Design review of the part built by this model. Coordinates are the model's own, in mm. A direction names the side the tool comes from. Give positions to 0.01 mm unless a question says otherwise; leave off trailing zeros. Write each loop counter-clockwise with the first axis right and the second up, starting at its lowest first coordinate (ties: lowest second). Pieces come first, ordered by that corner, then holes. Notation, with made-up numbers: (-32.75, 88) -> (-15.75, 88) arc R21 ccw to (-15.75, 110) -> close; hole circle Ø11 at (17.25, 76). An arc over 180 degrees is marked (long way). Write each question's results on one line, items separated by ' | '. Start each with the question number.
(1) To check wall thickness, follow probe 1 along Y at (x, z) = (81.5, 1.1); probe 2 along Y at (x, z) = (63.5, 2.95); probe 3 along X at (y, z) = (-4, 1.3) (3 decimals). State the ranges of each line that lie inside material, in increasing order.
(2) Take a section at A-A (y = 56). State the section outline as (x, z) points.
(3) Clearance check with flat-ended pins moving along their axes: pin 1 (1.2 mm diameter, centred on y = -0.5, z = 2, fed in from +X); pin 2 (2 mm diameter, centred on y = 26.5, z = 2, fed in from -X); pin 3 (1 mm diameter, centred on x = 41, y = 82.5, fed in from -Z); pin 4 (1.2 mm diameter, centred on x = 41.5, z = 2, fed in from -Y). State where each tip first meets the part, or that it passes through.
(4) Take a section at B-B (x = 53). State the section outline as (y, z) points, plus the area to 3 significant figures.
(5) For faces 1 (the face through (99.203, 19, 2)), 2 (the face through (-51.35, -42.92, 1.97)), list the 3-axis set-ups (+Z, -Z, +X, -X, +Y, -Y) from which the entire face can be reached by the end or side of a thin tool; tool diameter is ignored.
from build123d import *

# Parameters (mm, degrees)
F1_DEPTH = 4


with BuildPart() as f1:
    # F0 (on Top) → F1 (new body)
    with BuildSketch(Plane.XY):
        with BuildLine():
            Line((99.202662, 19.896773), (99.202662, 83.293949))
            ThreePointArc((99.202662, 83.293949), (102.639271, 102.736338), (83.237467, 99.077547))
            Line((83.237467, 99.077547), (19.823141, 99.077547))
            Line((19.823141, 99.077547), (-43.277989, 98.971398))
            ThreePointArc((-43.277989, 98.971398), (-62.685056, 102.776986), (-59.289763, 83.293949))
            Line((-59.289763, 83.293949), (-59.289763, 19.831447))
            Line((-59.289763, 19.831447), (-59.289763, -43.656712))
            ThreePointArc((-59.289763, -43.656712), (-62.72245, -63.080861), (-43.329186, -59.477778))
            Line((-43.329186, -59.477778), (83.190888, -59.221403))
            ThreePointArc((83.190888, -59.221403), (102.597955, -63.026992), (99.202662, -43.543955))
            Line((99.202662, -43.543955), (99.202662, 19.853222))
            Line((99.202662, 19.853222), (99.202662, 19.896773))
        make_face()
        with BuildLine():
            ThreePointArc((-42.274781, -54.475997), (-42.640605, -51.616895), (-43.677664, -48.927507))
            Line((-43.677664, -48.927507), (-24.605699, -29.855542))
            Line((-24.605699, -29.855542), (10.1243, -48.890038))
            Line((10.1243, -48.890038), (15.366075, -54.379034))
            Line((15.366075, -54.379034), (-42.274781, -54.475997))
        make_face(mode=Mode.SUBTRACT)
        with BuildLine():
            Line((-29.65462, -24.938536), (-48.66586, -43.949777))
            ThreePointArc((-48.66586, -43.949777), (-51.392585, -42.909613), (-54.289763, -42.558424))
            Line((-54.289763, -42.558424), (-54.289763, -42.539768))
            Line((-54.289763, -42.539768), (-54.289763, 15.079639))
            Line((-54.289763, 15.079639), (-48.808765, 9.87071))
            Line((-48.808765, 9.87071), (-29.65462, -24.938536))
        make_face(mode=Mode.SUBTRACT)
        with BuildLine():
            Line((20.115596, -48.890038), (-21.068434, -26.318277))
            Line((-21.068434, -26.318277), (0.785377, -4.464466))
            ThreePointArc((0.785377, -4.464466), (2.407493, -3.380602), (4.320911, -3))
            Line((4.320911, -3), (35.678927, -3))
            ThreePointArc((35.678927, -3), (37.592344, -3.380602), (39.214461, -4.464466))
            Line((39.214461, -4.464466), (61.034324, -26.284329))
            Line((61.034324, -26.284329), (20.115596, -48.890038))
        make_face(mode=Mode.SUBTRACT)
        with BuildLine():
            Line((64.568139, -29.818144), (83.594024, -48.844029))
            ThreePointArc((83.594024, -48.844029), (82.583872, -51.452044), (82.204858, -54.223054))
            Line((82.204858, -54.223054), (24.869697, -54.363046))
            Line((24.869697, -54.363046), (30.045989, -48.890038))
            Line((30.045989, -48.890038), (64.568139, -29.818144))
        make_face(mode=Mode.SUBTRACT)
        with BuildLine():
            Line((20.061165, 4.731285), (20.02865, 4.750027))
            ThreePointArc((20.02865, 4.750027), (20.061339, 4.750123), (20.094027, 4.75029))
            Line((20.094027, 4.75029), (20.061165, 4.731285))
        make_face(mode=Mode.SUBTRACT)
        with BuildLine():
            ThreePointArc((94.058243, -42.453536), (91.243307, -42.823298), (88.594024, -43.844029))
            Line((88.594024, -43.844029), (69.601331, -24.851336))
            Line((69.601331, -24.851336), (88.739303, 9.928519))
            Line((88.739303, 9.928519), (94.211702, 15.119198))
            Line((94.211702, 15.119198), (94.058243, -42.453536))
        make_face(mode=Mode.SUBTRACT)
        with BuildLine():
            Line((-8.87868, -3.300258), (-26.42517, -20.846748))
            Line((-26.42517, -20.846748), (-48.808765, 19.831447))
            Line((-48.808765, 19.831447), (-26.131123, 61.044022))
            Line((-26.131123, 61.044022), (-9.464466, 44.377365))
            ThreePointArc((-9.464466, 44.377365), (-8.380602, 42.755248), (-8, 40.841831))
            Line((-8, 40.841831), (-8, -1.178937))
            ThreePointArc((-8, -1.178937), (-8.228361, -2.326988), (-8.87868, -3.300258))
        make_face(mode=Mode.SUBTRACT)
        with BuildLine():
            Line((-48.681125, 83.594024), (-29.666657, 64.579555))
            Line((-29.666657, 64.579555), (-48.808765, 29.792184))
            Line((-48.808765, 29.792184), (-54.289763, 24.583255))
            Line((-54.289763, 24.583255), (-54.289763, 82.202662))
            ThreePointArc((-54.289763, 82.202662), (-51.400442, 82.555695), (-48.681125, 83.594024))
        make_face(mode=Mode.SUBTRACT)
        with BuildLine():
            Line((9.91038, 88.596564), (-24.61177, 69.524669))
            Line((-24.61177, 69.524669), (-43.681125, 88.594024))
            ThreePointArc((-43.681125, 88.594024), (-42.670973, 91.202039), (-42.291959, 93.973049))
            Line((-42.291959, 93.973049), (15.086671, 94.069572))
            Line((15.086671, 94.069572), (9.91038, 88.596564))
        make_face(mode=Mode.SUBTRACT)
        with BuildLine():
            Line((49.464466, 44.464466), (66.065797, 61.065797))
            Line((66.065797, 61.065797), (88.731457, 19.874997))
            Line((88.731457, 19.874997), (66.065797, -21.315802))
            Line((66.065797, -21.315802), (49.464466, -4.714471))
            ThreePointArc((49.464466, -4.714471), (48.380602, -3.092354), (48, -1.178937))
            Line((48, -1.178937), (48, 40.928932))
            ThreePointArc((48, 40.928932), (48.380602, 42.842349), (49.464466, 44.464466))
        make_face(mode=Mode.SUBTRACT)
        with BuildLine():
            Line((69.601331, 64.601331), (88.594024, 83.594024))
            ThreePointArc((88.594024, 83.594024), (91.243307, 82.573293), (94.058243, 82.203531))
            Line((94.058243, 82.203531), (94.211768, 24.606251))
            Line((94.211768, 24.606251), (88.743439, 29.813959))
            Line((88.743439, 29.813959), (69.601331, 64.601331))
        make_face(mode=Mode.SUBTRACT)
        with BuildLine():
            Line((19.840772, 88.596564), (61.024802, 66.024802))
            Line((61.024802, 66.024802), (39.464466, 44.464466))
            ThreePointArc((39.464466, 44.464466), (37.842349, 43.380602), (35.928932, 43))
            Line((35.928932, 43), (3.983967, 43))
            ThreePointArc((3.983967, 43), (2.07055, 43.380602), (0.448433, 44.464466))
            Line((0.448433, 44.464466), (-21.077956, 65.990855))
            Line((-21.077956, 65.990855), (19.840772, 88.596564))
        make_face(mode=Mode.SUBTRACT)
        with BuildLine():
            ThreePointArc((82.203158, 94.093463), (82.568962, 91.260377), (83.594024, 88.594024))
            Line((83.594024, 88.594024), (64.562068, 69.562068))
            Line((64.562068, 69.562068), (29.832068, 88.596564))
            Line((29.832068, 88.596564), (24.590293, 94.085559))
            Line((24.590293, 94.085559), (82.203158, 94.093463))
        make_face(mode=Mode.SUBTRACT)
    extrude(amount=F1_DEPTH)


solid = f1.part
Report:
1) probe 1: -59.22 to -54.22, -46.75 to -36.75, -3.23 to 6.73, 33.02 to 42.98, 76.5 to 86.5, 94.09 to 99.08 | probe 2: -59.26 to -54.27, -30.41 to -18.75, 58.5 to 70.14, 94.09 to 99.08 | probe 3: -59.29 to -54.29, -41.176 to -35.695, -9.578 to 1.321, 38.679 to 48.872, 75.594 to 81.075, 94.161 to 99.203
2) outline: (-59.29, 0) -> (-54.29, 0) -> (-54.29, 4) -> (-59.29, 4) -> close; (-34.39, 0) -> (-28.91, 0) -> (-28.91, 4) -> (-34.39, 4) -> close; (-21.09, 0) -> (-11.09, 0) -> (-11.09, 4) -> (-21.09, 4) -> close; (51, 0) -> (61, 0) -> (61, 4) -> (51, 4) -> close; (68.85, 0) -> (74.33, 0) -> (74.33, 4) -> (68.85, 4) -> close; (94.13, 0) -> (99.2, 0) -> (99.2, 4) -> (94.13, 4) -> close
3) pin 1: x = 99.2 | pin 2: x = -59.29 | pin 3: z = 0 | pin 4: y = -59.31
4) outline: (-59.28, 0) -> (-54.29, 0) -> (-54.29, 4) -> (-59.28, 4) -> close; (-36.21, 0) -> (-30.72, 0) -> (-30.72, 4) -> (-36.21, 4) -> close; (-18.25, 0) -> (-8.25, 0) -> (-8.25, 4) -> (-18.25, 4) -> close; (48, 0) -> (58, 0) -> (58, 4) -> (48, 4) -> close; (70.42, 0) -> (75.9, 0) -> (75.9, 4) -> (70.42, 4) -> close; (94.09, 0) -> (99.08, 0) -> (99.08, 4) -> (94.09, 4) -> close | area: 164 mm2
5) face 1: +Z, -Z, +X | face 2: +Z, -Z
